from build123d import *

# Parameters (mm, degrees)
SKETCH2_W                      = 18
SKETCH2_H                      = 14
BOSS_EXTRUDE1_DEPTH            = 37
SKETCH3_R                      = 5
CUT_EXTRUDE1_DEPTH             = 15
M3X0_5_TAPPED_HOLE1_AT_2_COUNT = 2
M3X0_5_TAPPED_HOLE1_AT_2_PITCH = 8
M3X0_5_TAPPED_HOLE1_AT_3_COUNT = 2
M3X0_5_TAPPED_HOLE1_AT_3_PITCH = 15.264337522
M3X0_5_TAPPED_HOLE1_AT_4_COUNT = 2
M3X0_5_TAPPED_HOLE1_AT_4_PITCH = 13


with BuildPart() as part:
    # Sketch2 → Boss-Extrude1 (new body)
    with BuildSketch(Plane(origin=(0, 0, 0), x_dir=(1, 0, 0), z_dir=(0, 1, 0))):
        Rectangle(SKETCH2_W, SKETCH2_H)
    extrude(amount=BOSS_EXTRUDE1_DEPTH)

    # Sketch3 → Cut-Extrude1 (cut, through all)
    with BuildSketch(Plane.XY.offset(7)):
        with Locations((0, 26)):
            Circle(SKETCH3_R)
        with Locations((0, 11)):
            Circle(SKETCH3_R)
    extrude(amount=-CUT_EXTRUDE1_DEPTH, mode=Mode.SUBTRACT)

    # Sketch5 → M3x0.5 Tapped Hole1 (revolve, cut)
    with BuildSketch(Plane(origin=(-9, 17.5, -4), x_dir=(0, 0, 1), z_dir=(0, 1, 0))):
        Polygon((0, 0), (0, 6.251075774), (1.25, 5.5), (1.25, 0), align=None)
    m3x0_5_tapped_hole1 = revolve(axis=Axis((-15.35, 17.5, -4), (1, 0, 0)), mode=Mode.SUBTRACT)

    # M3x0.5 Tapped Hole1 at 2: M3x0.5 Tapped Hole1 ×2
    with Locations(*[(0, 0, i * M3X0_5_TAPPED_HOLE1_AT_2_PITCH) for i in range(1, M3X0_5_TAPPED_HOLE1_AT_2_COUNT)]):
        add(m3x0_5_tapped_hole1, mode=Mode.SUBTRACT)

    # M3x0.5 Tapped Hole1 at 3: M3x0.5 Tapped Hole1 ×2
    with Locations(*[Vector(0, -0.851658317, 0.524097426) * (i * M3X0_5_TAPPED_HOLE1_AT_3_PITCH) for i in range(1, M3X0_5_TAPPED_HOLE1_AT_3_COUNT)]):
        add(m3x0_5_tapped_hole1, mode=Mode.SUBTRACT)

    # M3x0.5 Tapped Hole1 at 4: M3x0.5 Tapped Hole1 ×2
    with Locations(*[(0, -i * M3X0_5_TAPPED_HOLE1_AT_4_PITCH, 0) for i in range(1, M3X0_5_TAPPED_HOLE1_AT_4_COUNT)]):
        add(m3x0_5_tapped_hole1, mode=Mode.SUBTRACT)

    # Mirror1: M3x0.5 Tapped Hole1 across plane
    add(m3x0_5_tapped_hole1.mirror(Plane(origin=(0, 0, 0), x_dir=(0, 0, 1), z_dir=(1, 0, 0))), mode=Mode.SUBTRACT)

    # Mirror1 copy 1 sketch → Mirror1 copy 1 (revolve, cut)
    with BuildSketch(Plane(origin=(9, 17.5, 4), x_dir=(0, 0, 1), z_dir=(0, 1, 0))):
        Polygon((0, 0), (0, -6.251075774), (1.25, -5.5), (1.25, 0), align=None)
    revolve(axis=Axis((15.35, 17.5, 4), (1, 0, 0)), mode=Mode.SUBTRACT)

    # Mirror1 copy 2 sketch → Mirror1 copy 2 (revolve, cut)
    with BuildSketch(Plane(origin=(9, 4.5, 4), x_dir=(0, 0, 1), z_dir=(0, 1, 0))):
        Polygon((0, 0), (0, -6.251075774), (1.25, -5.5), (1.25, 0), align=None)
    revolve(axis=Axis((15.35, 4.5, 4), (1, 0, 0)), mode=Mode.SUBTRACT)

    # Mirror1 copy 3 sketch → Mirror1 copy 3 (revolve, cut)
    with BuildSketch(Plane(origin=(9, 4.5, -4), x_dir=(0, 0, 1), z_dir=(0, 1, 0))):
        Polygon((0, 0), (0, -6.251075774), (1.25, -5.5), (1.25, 0), align=None)
    revolve(axis=Axis((15.35, 4.5, -4), (1, 0, 0)), mode=Mode.SUBTRACT)


solid = part.part
Can you work these out from the model? Positions are in its coordinate system, mm. A direction names the side the tool comes from. Give positions to 0.01 mm unless a question says otherwise; leave off trailing zeros. Order: outer loops, then holes, each group sorted by start corner. A loop starts at its lowest first (then second) coordinate and runs counter-clockwise, first axis right, second up. Notation, with made-up numbers: M 6.5,40.25 L 26.5,40.25 A15 ccw 26.5,51.25 Z; hole C 28,26.5 d9. An arc over 180 degrees is marked long. Use a Markdown table: item, result. Add a question column.
Item 1: Suppose I cut it at A-A (x = 0). List the corners of the cut face in (y, z) for me.
Item 2: For faces 4 (the cylindrical face through (6.288, 16.655, -4.921)), 5 (the flat face through (-9, 18, 0)), 6 (the cylindrical face through (-6.29, 5.72, -4.27)), which set-ups out of +Z, -Z, +X, -X, +Y, -Y let a thin tool reach every point of the face, with its end or its side?
Item 3: Suppose I cut it at B-B (y = 14). List the corners of the cut face in (x, z) for me, then the cut area to 3 significant figures.
Item 4: Suppose I cut it at C-C (z = 1.25). List the corners of the cut face in (x, y) for me, then the cut area to 3 significant figures.
Item 5: If I drill on L1, parallel to Z at x = 5, y = 17.5; L2, parallel to Y at x = 6.3, z = -4; L3, parallel to Y at x = 0.5, z = 3.75, over which ranges is the centre line in solid material (lowest first)? Write a range as [from, to].
Item 6: We'd pull the mould along Y, two halves only. Please class faces 1 (the flat face through (0, 37, 0)), 2 (the flat face through (9, 18, 0)), 3 (the conical face through (2.88, 4.35, -4.16)): +Y half, -Y half, draft (parallel to the pull), parting line (faces both ways), or undercut.
Item 7: Will these pins go through, and if not, where does the flat tip stop? pin 1 (8 mm diameter, centred on x = -1, y = 29, fed in from +Z); pin 2 (2 mm diameter, centred on y = 17.5, z = -4, fed in from +X); pin 3 (2 mm diameter, centred on y = 4.5, z = 4, fed in from -X).
Item 8: Suppose I cut it at D-D (x = -7.5). List the corners of the cut face in (y, z) for me.
Answer sheet:
| question | item | result |
|---|---|---|
| 1 | outline | M 0,-7 L 6,-7 L 6,7 L 0,7 Z; M 16,-7 L 21,-7 L 21,7 L 16,7 Z; M 31,-7 L 37,-7 L 37,7 L 31,7 Z |
| 2 | face 4 | +X |
| 2 | face 5 | +Z, -Z, -X, +Y, -Y |
| 2 | face 6 | -X |
| 3 | outline | M -9,-7 L -4,-7 L -4,7 L -9,7 Z; M 4,-7 L 9,-7 L 9,7 L 4,7 Z |
| 3 | area | 140 mm² |
| 4 | outline | M -9,0 L 9,0 L 9,37 L -9,37 Z; hole C 0,11 d10; hole C 0,26 d10 |
| 4 | area | 509 mm² |
| 5 | L1 | z = [-7, -5.25], [-2.75, 2.75], [5.25, 7] |
| 5 | L2 | y = [0, 3.25], [5.75, 16.25], [18.75, 37] |
| 5 | L3 | y = [0, 6.03], [15.97, 21.03], [30.97, 37] |
| 6 | face 1 | +Y half |
| 6 | face 2 | draft |
| 6 | face 3 | undercut |
| 7 | pin 1 | stops at z = 7 |
| 7 | pin 2 | stops at x = 3.35 |
| 7 | pin 3 | stops at x = -3.35 |
| 8 | outline | M 0,-7 L 37,-7 L 37,7 L 0,7 Z; hole C 4.5,-4 d2.5; hole C 4.5,4 d2.5; hole C 17.5,-4 d2.5; hole C 17.5,4 d2.5 |
